Could you check a few things on this drawing? It's one solid part, dimensions in mm from its lowest x, y, z. Coordinates: 2 decimals unless noted, no trailing zeros. Order: outer loops, then holes, each group sorted by start corner. A loop starts at its lowest first (then second) coordinate and runs counter-clockwise, first axis right, second up.
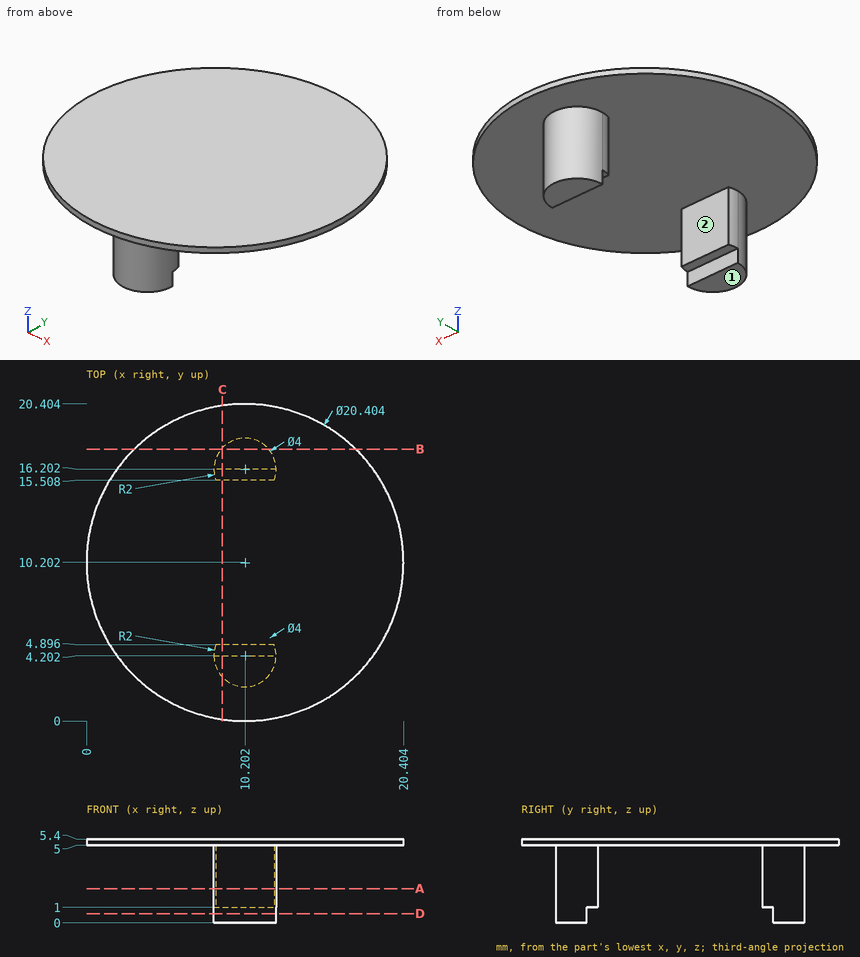
Item 1: I need wall thicknesses on line 1 (Z direction, x = 10, y = 14.25); line 2 (Y direction, x = 11, z = 0.6) (1 decimal); line 3 (Y direction, x = 11.5, z = 4.9) (1 decimal). Which ranges of each line are inside material? Lowest first, please.
Item 2: Suppose I cut it at A-A (z = 2.2). List the corners of the cut face in (x, y) for me (1 decimal), and give its area (3 significant figures).
Item 3: Thinking about a two-plate mould opening in Y: for the marked faces 1 and 2, which applies, +Y half, -Y half, draft (parallel to the pull), parting line (faces both ways), or undercut?
Item 4: For pin 1 Ø0.8 at (x, y) = (10, 16) entering from -Z; pin 2 Ø1.9 at (x, z) = (10.5, 3) entering from -Y; pin 3 Ø1 at (x, z) = (13.5, 5) entering from +Y; pin 4 Ø1.1 at (x, z) = (10.5, 2) entering from +Y, each with a flat end and sliding along its axis, tell me the tip position at first contact or that it passes through.
Item 5: Suppose I cut it at D-D (z = 0.6). List the corners of the cut face in (x, y) for me.
Item 6: Suppose I cut it at B-B (y = 17.5). List the corners of the cut face in (x, z) for me.
Item 7: Suppose I cut it at C-C (x = 8.75). List the corners of the cut face in (y, z) for me (1 decimal).
Geometry results:
1. line 1: z = 5 to 5.4
1. line 2: y = 2.4 to 4.2, 16.2 to 18
1. line 3: y = 2.7 to 4.9, 15.5 to 17.7
2. outline: (8.3, 4.9) arc R2 ccw (long way) to (12.1, 4.9) - close; (8.3, 15.5) - (12.1, 15.5) arc R2 ccw (long way) to start
2. area: 18.0 mm2
3. face 1: draft
3. face 2: undercut
4. pin 1: stops at z = 0
4. pin 2: stops at y = 2.2
4. pin 3: stops at y = 20.01
4. pin 4: stops at y = 18.2
5. outline: (8.2, 4.2) arc R2 ccw to (12.2, 4.2) - close; (8.2, 16.2) - (12.2, 16.2) arc R2 ccw to start
6. outline: (3.07, 5) - (8.68, 5) - (8.68, 0) - (11.72, 0) - (11.72, 5) - (17.33, 5) - (17.33, 5.4) - (3.07, 5.4) - close
7. outline: (0.1, 5) - (2.8, 5) - (2.8, 0) - (4.2, 0) - (4.2, 1) - (4.9, 1) - (4.9, 5) - (15.5, 5) - (15.5, 1) - (16.2, 1) - (16.2, 0) - (17.6, 0) - (17.6, 5) - (20.3, 5) - (20.3, 5.4) - (0.1, 5.4) - close
